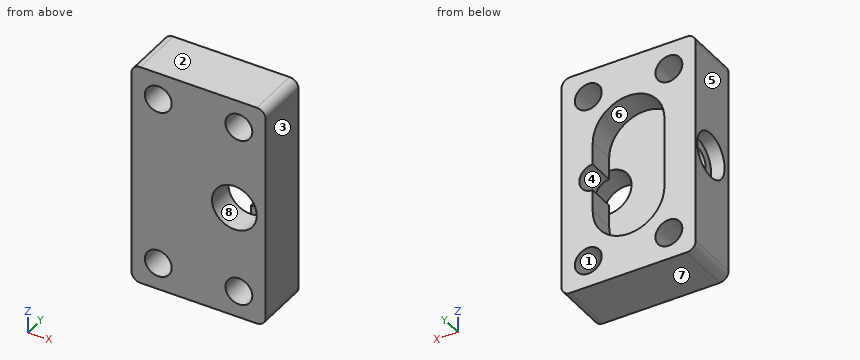
from build123d import *

# Parameters (mm, degrees)
SKETCH1_W                 = 15
SKETCH1_H                 = 25
BOSS_EXTRUDE1_DEPTH       = 6
CUT_EXTRUDE1_DEPTH        = 3
SKETCH3_R                 = 1.5
CUT_EXTRUDE2_DEPTH        = 16.76388277
SKETCH4_R                 = 2.5
CUT_EXTRUDE3_DEPTH        = 3
F_3_0MM_DOWEL_HOLE1_D     = 3
F_3_0MM_DOWEL_HOLE1_DEPTH = 3
F_3_0MM_DOWEL_HOLE1_TIP   = 0.901290929
SKETCH7_R                 = 2.5
CUT_EXTRUDE4_DEPTH        = 1.5
FILLET1_R                 = 1


with BuildPart() as part:
    # Sketch1 → Boss-Extrude1 (new body)
    with BuildSketch(Plane(origin=(0, 0, 0), x_dir=(1, 0, 0), z_dir=(0, 1, 0))):
        Rectangle(SKETCH1_W, SKETCH1_H)
    extrude(amount=BOSS_EXTRUDE1_DEPTH)

    # Sketch2 → Cut-Extrude1 (cut)
    with BuildSketch(Plane(origin=(0, 6, 0), x_dir=(1, 0, 0), z_dir=(0, 1, 0))):
        with BuildLine():
            Line((4, 4), (4, 1.5))
            ThreePointArc((4, 1.5), (5.5, 0), (4, -1.5))
            Line((4, -1.5), (4, -4))
            ThreePointArc((4, -4), (0, -8), (-4, -4))
            Line((-4, -4), (-4, 4))
            ThreePointArc((-4, 4), (0, 8), (4, 4))
        make_face()
    extrude(amount=-CUT_EXTRUDE1_DEPTH, mode=Mode.SUBTRACT)

    # Sketch3 → Cut-Extrude2 (cut, through all)
    with BuildSketch(Plane(origin=(0, 6, 0), x_dir=(1, 0, 0), z_dir=(0, 1, 0))):
        with Locations(Location((-4.5, 9.5, 0), (0, 0, 270))):
            Circle(SKETCH3_R)
        with Locations(Location((4.5, 9.5, 0), (0, 0, 270))):
            Circle(SKETCH3_R)
        with Locations(Location((-4.5, -9.5, 0), (0, 0, 270))):
            Circle(SKETCH3_R)
        with Locations(Location((4.5, -9.5, 0), (0, 0, 270))):
            Circle(SKETCH3_R)
    extrude(amount=-CUT_EXTRUDE2_DEPTH, mode=Mode.SUBTRACT)

    # Sketch4 → Cut-Extrude3 (cut)
    with BuildSketch(Plane.XZ):
        with Locations(Location((4, 0, 0), (0, 0, 270))):
            Circle(SKETCH4_R)
    extrude(amount=-CUT_EXTRUDE3_DEPTH, mode=Mode.SUBTRACT)

    # Ø3.0mm Dowel Hole1
    with Locations(Plane.ZY.offset(7.5)):
        with Locations((0, 3.230523086)):
            Hole(F_3_0MM_DOWEL_HOLE1_D / 2, depth=F_3_0MM_DOWEL_HOLE1_DEPTH)
            with Locations((0, 0, -(F_3_0MM_DOWEL_HOLE1_DEPTH + F_3_0MM_DOWEL_HOLE1_TIP / 2))):  # 118° drill point
                Cone(0, F_3_0MM_DOWEL_HOLE1_D / 2, F_3_0MM_DOWEL_HOLE1_TIP, mode=Mode.SUBTRACT)

    # Sketch7 → Cut-Extrude4 (cut)
    with BuildSketch(Plane.ZY.offset(7.5)):
        with Locations((0, 3.230523086)):
            Circle(SKETCH7_R)
    extrude(amount=-CUT_EXTRUDE4_DEPTH, mode=Mode.SUBTRACT)

    # Fillet1
    fillet1_edges = [part.edges().sort_by_distance(p)[0] for p in [
        (7.5, 3, 12.5),
        (-7.5, 3, 12.5),
        (-7.5, 3, -12.5),
        (7.5, 3, -12.5),
    ]]
    fillet(fillet1_edges, radius=FILLET1_R)


solid = part.part
CAD build for the part. Positions are in the model's coordinates, mm. Face numbers are marked on the shaded views. A direction names the side the tool comes from. Give positions to 0.01 mm unless a question says otherwise; leave off trailing zeros. Order: outer loops, then holes, each group sorted by start corner. A loop starts at its lowest first (then second) coordinate and runs counter-clockwise, first axis right, second up. Notation, with made-up numbers: (68, 64.5) -> (123, 64.5) arc R24 cw to (123, 81.5) -> close; hole circle Ø8 at (5.5, 6.25). An arc over 180 degrees is marked (long way). Return JSON: item names as keys, results as strings.
Q1. Saw through at C-C (x = -5.25). Write the cut outline in (y, z), then the cut area to 3 significant figures.
Working result:
{"outline": "(0, -12.5) -> (6, -12.5) -> (6, -10.8) -> (0, -10.8) -> close; (0, -8.2) -> (6, -8.2) -> (6, 8.2) -> (0, 8.2) -> close; (0, 10.8) -> (6, 10.8) -> (6, 12.5) -> (0, 12.5) -> close; hole circle Ø3 at (3.23, 0)", "area": "112 mm²"}
Q2. Saw through at B-B (x = 4.5). Write the cut outline in (y, z), then the cut area to 3 significant figures.
Working result:
{"outline": "(0, -12.5) -> (6, -12.5) -> (6, -11) -> (0, -11) -> close; (0, -8) -> (6, -8) -> (6, -1.41) -> (3, -1.41) -> (3, -2.45) -> (0, -2.45) -> close; (0, 2.45) -> (3, 2.45) -> (3, 1.41) -> (6, 1.41) -> (6, 8) -> (0, 8) -> close; (0, 11) -> (6, 11) -> (6, 12.5) -> (0, 12.5) -> close", "area": "90.8 mm²"}
Q3. Saw through at A-A (z = -9.5). Write the cut outline in (x, y), then the cut area to 3 significant figures.
Working result:
{"outline": "(-7.5, 0) -> (-6, 0) -> (-6, 6) -> (-7.5, 6) -> close; (-3, 0) -> (3, 0) -> (3, 6) -> (-3, 6) -> close; (6, 0) -> (7.5, 0) -> (7.5, 6) -> (6, 6) -> close", "area": "54.0 mm²"}
Q4. Flat gauge pins, fed straight in: pin 1 (4 mm diameter, centred on x = 0.5, z = -4, fed in from +Y); pin 2 (2.5 mm diameter, centred on x = -4.5, z = -9.5, fed in from -Y); pin 3 (2 mm diameter, centred on x = 5, z = 0.5, fed in from -Y). Where does each tip first touch, or does it go through?
Working result:
{"pin 1": "y = 3", "pin 2": "through", "pin 3": "y = 3"}
Q5. Mould opens along Z. For the marked faces 1, 2 and 3 say: pulls with the +Z half, pulls with the -Z half, needs draft (parallel to the pull), parting line crosses it, or undercut.
Working result:
{"face 1": "undercut", "face 2": "pulls with the +Z half", "face 3": "needs draft"}
Q6. Saw through at D-D (y = 1.05). Write the cut outline in (x, z).
Working result:
{"outline": "(-7.5, -11.5) arc R1 ccw to (-6.5, -12.5) -> (6.5, -12.5) arc R1 ccw to (7.5, -11.5) -> (7.5, 11.5) arc R1 ccw to (6.5, 12.5) -> (-6.5, 12.5) arc R1 ccw to (-7.5, 11.5) -> (-7.5, 1.22) -> (-6, 1.22) -> (-6, -1.22) -> (-7.5, -1.22) -> close; hole circle Ø3 at (-4.5, -9.5); hole circle Ø3 at (-4.5, 9.5); hole circle Ø5 at (4, 0); hole circle Ø3 at (4.5, -9.5); hole circle Ø3 at (4.5, 9.5)"}
Q7. Drill centre lines: line 1 (X direction, y = 1.65, z = 9.5); line 2 (Y direction, x = -4.9, z = 0); line 3 (X direction, y = 1.5, z = 0). Where is each one in solid material? Low to high.
Working result:
{"line 1": "-7.5 to -6, -3 to 3, 6 to 7.5", "line 2": "0 to 1.73, 4.73 to 6", "line 3": "-6 to 1.5, 6.5 to 7.5"}
Q8. Which spindle directions (+Z, -Z, +X, -X, +Y, -Y) get a long thin tool onto all of the face, cutting with end or side? Do the marked faces 4, 5, 6, 7 and 8. Say none if no direction does.
Working result:
{"face 4": "+Y, -Y", "face 5": "+Z, -Z, -X, +Y, -Y", "face 6": "+Y", "face 7": "-Z, +X, -X, +Y, -Y", "face 8": "-Y"}
